Verification items for the finished model (mm, model axes). Coordinates: 2 decimals unless noted, no trailing zeros. Loops run counter-clockwise (first coordinate to the right, second up) from the corner with the lowest first, then second, coordinate; pieces in that order, holes last. Notation, with made-up numbers: (6.5, -7.5) -> (20.5, -7.5) arc R12 ccw to (20.5, 7.5) -> close; hole circle Ø4 at (1.25, 36). An arc over 180 degrees is marked (long way). Write item = value, one per line.
```python
from build123d import *

# Parameters (mm, degrees)
SKETCH1_W                   = 43.18
SKETCH1_H                   = 30.48
SKETCH1_R                   = 1.0541
BOSS_EXTRUDE1_DEPTH         = 1.5875
CAMERA_CUTS_REACH           = 39.386
SKETCH5_W                   = 9
SKETCH5_H                   = 2.93
SKETCH5_W_2                 = 8.509
SKETCH5_H_2                 = 4.826
SKETCH5_W_3                 = 3.175
SKETCH5_H_3                 = 2.6162
SKETCH5_W_4                 = 4.22
SKETCH5_H_4                 = 7.75
SKETCH6_W                   = 5.0927
SKETCH6_H                   = 10.1092
WEIGHT_REDUCTION_CUTS_DEPTH = 2.54
ATTACHMENT_CUTS_REACH       = 39.386
SKETCH7_W                   = 1.5875
SKETCH7_H                   = 1.3208
FILLET8_R                   = 0.762


with BuildPart() as part:
    # Sketch1 → Boss-Extrude1 (new body)
    with BuildSketch(Plane.XY):
        with Locations((0, 15.24)):
            Rectangle(SKETCH1_W, SKETCH1_H)
        with Locations((17.48282, 2.159)):
            Circle(SKETCH1_R, mode=Mode.SUBTRACT)
        with Locations((17.48282, 23.749)):
            Circle(SKETCH1_R, mode=Mode.SUBTRACT)
        with Locations((-19.431, 2.159)):
            Circle(SKETCH1_R, mode=Mode.SUBTRACT)
        with Locations((-19.431, 23.749)):
            Circle(SKETCH1_R, mode=Mode.SUBTRACT)
    extrude(amount=BOSS_EXTRUDE1_DEPTH)

    # Sketch5 → Camera Cuts (cut, up to next)
    with BuildSketch(Plane.XY.offset(1.5875), mode=Mode.PRIVATE) as camera_cuts_sk1:
        with Locations((-12.151, 22.413)):
            Rectangle(SKETCH5_W, SKETCH5_H)
    camera_cuts_tool1 = extrude(camera_cuts_sk1.sketch, amount=-CAMERA_CUTS_REACH, mode=Mode.PRIVATE) & part.part
    # Sketch5 → Camera Cuts (cut, up to next)
    with BuildSketch(Plane.XY.offset(1.5875), mode=Mode.PRIVATE) as camera_cuts_sk2:
        with Locations((1.9341, 22.597)):
            Rectangle(SKETCH5_W_2, SKETCH5_H_2)
    camera_cuts_tool2 = extrude(camera_cuts_sk2.sketch, amount=-CAMERA_CUTS_REACH, mode=Mode.PRIVATE) & part.part
    # Sketch5 → Camera Cuts (cut, up to next)
    with BuildSketch(Plane.XY.offset(1.5875), mode=Mode.PRIVATE) as camera_cuts_sk3:
        with Locations((11.5861, 23.7019)):
            Rectangle(SKETCH5_W_3, SKETCH5_H_3)
    camera_cuts_tool3 = extrude(camera_cuts_sk3.sketch, amount=-CAMERA_CUTS_REACH, mode=Mode.PRIVATE) & part.part
    # Sketch5 → Camera Cuts (cut, up to next)
    with BuildSketch(Plane.XY.offset(1.5875), mode=Mode.PRIVATE) as camera_cuts_sk4:
        with Locations((16.5326, 13.0085)):
            Rectangle(SKETCH5_W_4, SKETCH5_H_4)
    camera_cuts_tool4 = extrude(camera_cuts_sk4.sketch, amount=-CAMERA_CUTS_REACH, mode=Mode.PRIVATE) & part.part
    add(camera_cuts_tool1.solids().sort_by_distance((-12.151, 22.413, 1.5875))[0], mode=Mode.SUBTRACT)
    add(camera_cuts_tool2.solids().sort_by_distance((1.9341, 22.597, 1.5875))[0], mode=Mode.SUBTRACT)
    add(camera_cuts_tool3.solids().sort_by_distance((11.5861, 23.7019, 1.5875))[0], mode=Mode.SUBTRACT)
    add(camera_cuts_tool4.solids().sort_by_distance((16.5326, 13.0085, 1.5875))[0], mode=Mode.SUBTRACT)

    # Sketch6 → Weight Reduction Cuts (cut)
    with BuildSketch(Plane.XY.offset(1.5875)):
        Polygon((9.163785799, 2.54), (0.61365, 8.540457725), (-7.936485799, 2.54), align=None)
        Polygon((2.824464201, 10.092), (11.3746, 4.091542275), (11.3746, 16.092457725), align=None)
        Polygon((-7.936485799, 17.644), (0.61365, 11.643542275), (9.163785799, 17.644), align=None)
        Polygon((-10.1473, 4.091542275), (-1.597164201, 10.092), (-10.1473, 16.092457725), align=None)
        with Locations((-16.50365, 11.479427373)):
            Rectangle(SKETCH6_W, SKETCH6_H)
    extrude(amount=-WEIGHT_REDUCTION_CUTS_DEPTH, mode=Mode.SUBTRACT)

    # Sketch7 → Attachment Cuts (cut, up to next)
    with BuildSketch(Plane(origin=(0, 0, 0), x_dir=(-1, 0, 0), z_dir=(0, 0, -1)), mode=Mode.PRIVATE) as attachment_cuts_sk1:
        with Locations((13.98905, 27.405227373)):
            Rectangle(SKETCH7_W, SKETCH7_H)
    attachment_cuts_tool1 = extrude(attachment_cuts_sk1.sketch, amount=-ATTACHMENT_CUTS_REACH, mode=Mode.PRIVATE) & part.part
    # Sketch7 → Attachment Cuts (cut, up to next)
    with BuildSketch(Plane(origin=(0, 0, 0), x_dir=(-1, 0, 0), z_dir=(0, 0, -1)), mode=Mode.PRIVATE) as attachment_cuts_sk2:
        with Locations((13.98905, 18.464427373)):
            Rectangle(SKETCH7_W, SKETCH7_H)
    attachment_cuts_tool2 = extrude(attachment_cuts_sk2.sketch, amount=-ATTACHMENT_CUTS_REACH, mode=Mode.PRIVATE) & part.part
    # Sketch7 → Attachment Cuts (cut, up to next)
    with BuildSketch(Plane(origin=(0, 0, 0), x_dir=(-1, 0, 0), z_dir=(0, 0, -1)), mode=Mode.PRIVATE) as attachment_cuts_sk3:
        with Locations((13.98905, 4.494427373)):
            Rectangle(SKETCH7_W, SKETCH7_H)
    attachment_cuts_tool3 = extrude(attachment_cuts_sk3.sketch, amount=-ATTACHMENT_CUTS_REACH, mode=Mode.PRIVATE) & part.part
    # Sketch7 → Attachment Cuts (cut, up to next)
    with BuildSketch(Plane(origin=(0, 0, 0), x_dir=(-1, 0, 0), z_dir=(0, 0, -1)), mode=Mode.PRIVATE) as attachment_cuts_sk4:
        with Locations((-19.78025, 4.494427373)):
            Rectangle(SKETCH7_W, SKETCH7_H)
    attachment_cuts_tool4 = extrude(attachment_cuts_sk4.sketch, amount=-ATTACHMENT_CUTS_REACH, mode=Mode.PRIVATE) & part.part
    # Sketch7 → Attachment Cuts (cut, up to next)
    with BuildSketch(Plane(origin=(0, 0, 0), x_dir=(-1, 0, 0), z_dir=(0, 0, -1)), mode=Mode.PRIVATE) as attachment_cuts_sk5:
        with Locations((-19.78025, 21.004427373)):
            Rectangle(SKETCH7_W, SKETCH7_H)
    attachment_cuts_tool5 = extrude(attachment_cuts_sk5.sketch, amount=-ATTACHMENT_CUTS_REACH, mode=Mode.PRIVATE) & part.part
    # Sketch7 → Attachment Cuts (cut, up to next)
    with BuildSketch(Plane(origin=(0, 0, 0), x_dir=(-1, 0, 0), z_dir=(0, 0, -1)), mode=Mode.PRIVATE) as attachment_cuts_sk6:
        with Locations((-19.78025, 27.405227373)):
            Rectangle(SKETCH7_W, SKETCH7_H)
    attachment_cuts_tool6 = extrude(attachment_cuts_sk6.sketch, amount=-ATTACHMENT_CUTS_REACH, mode=Mode.PRIVATE) & part.part
    add(attachment_cuts_tool1.solids().sort_by_distance((-13.98905, 27.405227, 0))[0], mode=Mode.SUBTRACT)
    add(attachment_cuts_tool2.solids().sort_by_distance((-13.98905, 18.464427, 0))[0], mode=Mode.SUBTRACT)
    add(attachment_cuts_tool3.solids().sort_by_distance((-13.98905, 4.494427, 0))[0], mode=Mode.SUBTRACT)
    add(attachment_cuts_tool4.solids().sort_by_distance((19.78025, 4.494427, 0))[0], mode=Mode.SUBTRACT)
    add(attachment_cuts_tool5.solids().sort_by_distance((19.78025, 21.004427, 0))[0], mode=Mode.SUBTRACT)
    add(attachment_cuts_tool6.solids().sort_by_distance((19.78025, 27.405227, 0))[0], mode=Mode.SUBTRACT)

    # Fillet8
    fillet8_edges = [part.edges().sort_by_distance(p)[0] for p in [
        (9.163785799, 17.644, 0.79375),
        (0.61365, 11.643542275, 0.79375),
        (-7.936485799, 17.644, 0.79375),
        (-1.597164201, 10.092, 0.79375),
        (-10.1473, 4.091542275, 0.79375),
        (-10.1473, 16.092457725, 0.79375),
        (-13.9573, 6.424827373, 0.79375),
        (-19.05, 6.424827373, 0.79375),
        (-19.05, 16.534027373, 0.79375),
        (-13.9573, 16.534027373, 0.79375),
        (0.61365, 8.540457725, 0.79375),
        (9.163785799, 2.54, 0.79375),
        (-7.936485799, 2.54, 0.79375),
        (11.3746, 16.092457725, 0.79375),
        (11.3746, 4.091542275, 0.79375),
        (2.824464201, 10.092, 0.79375),
    ]]
    fillet(fillet8_edges, radius=FILLET8_R)


solid = part.part
```
1) Material ranges on line 1 (Y direction, x = 20, z = 0.6); line 2 (X direction, y = 10, z = 0.55); line 3 (X direction, y = 27.5, z = 0.55), recorded low to high.
Ans:
line_1 = 0 to 3.83, 5.15 to 20.34, 21.66 to 26.74, 28.07 to 30.48
line_2 = -21.59 to -19.05, -13.96 to -10.15, -2.17 to 3.39, 11.37 to 14.42, 18.64 to 21.59
line_3 = -21.59 to -14.78, -13.2 to 18.99, 20.57 to 21.59
2) Sectioned sample at C-C, the plane x = 5. Record the cut outline in (y, z).
Ans:
outline = (0, 0) -> (2.54, 0) -> (2.54, 1.59) -> (0, 1.59) -> close; (5.46, 0) -> (8.57, 0) -> (8.57, 1.59) -> (5.46, 1.59) -> close; (11.62, 0) -> (14.72, 0) -> (14.72, 1.59) -> (11.62, 1.59) -> close; (17.64, 0) -> (20.18, 0) -> (20.18, 1.59) -> (17.64, 1.59) -> close; (25.01, 0) -> (30.48, 0) -> (30.48, 1.59) -> (25.01, 1.59) -> close
3) Sectioned sample at B-B, the plane y = 18.5. Record the cut outline in (x, z), plus the area to 3 significant figures.
Ans:
outline = (-21.59, 0) -> (-14.78, 0) -> (-14.78, 1.59) -> (-21.59, 1.59) -> close; (-13.2, 0) -> (21.59, 0) -> (21.59, 1.59) -> (-13.2, 1.59) -> close
area = 66.0 mm2
4) Release check for a two-part mould opening along X. For faces 1 (the face through (21.59, 15, 1)), 2 (the face through (0, 19, 1.588)), 3 (the face through (20, 28.066, 1)) record: pulls with the +X half, pulls with the -X half, needs draft (parallel to the pull), parting line crosses it, or undercut.
Ans:
face_1 = pulls with the +X half
face_2 = needs draft
face_3 = undercut
5) Sectioned sample at D-D, the plane y = 13. Record the cut outline in (x, z).
Ans:
outline = (-21.59, 0) -> (-19.05, 0) -> (-19.05, 1.59) -> (-21.59, 1.59) -> close; (-13.96, 0) -> (-10.15, 0) -> (-10.15, 1.59) -> (-13.96, 1.59) -> close; (-5.74, 0) -> (-1.32, 0) -> (-1.32, 1.59) -> (-5.74, 1.59) -> close; (2.55, 0) -> (6.97, 0) -> (6.97, 1.59) -> (2.55, 1.59) -> close; (11.37, 0) -> (14.42, 0) -> (14.42, 1.59) -> (11.37, 1.59) -> close; (18.64, 0) -> (21.59, 0) -> (21.59, 1.59) -> (18.64, 1.59) -> close
6) Sectioned sample at A-A, the plane x = -15.5. Record the cut outline in (y, z), plus the area to 3 significant figures.
Ans:
outline = (0, 0) -> (6.42, 0) -> (6.42, 1.59) -> (0, 1.59) -> close; (16.53, 0) -> (20.95, 0) -> (20.95, 1.59) -> (16.53, 1.59) -> close; (23.88, 0) -> (30.48, 0) -> (30.48, 1.59) -> (23.88, 1.59) -> close
area = 27.7 mm2
